```python
from build123d import *

# Parameters (mm, degrees)
SKETCH105_W     = 290
SKETCH105_H     = 290
PAD053_DEPTH    = 10
SKETCH106_R     = 5
SKETCH106_R_2   = 2.5
POCKET048_DEPTH = 10.001
SKETCH107_W     = 270
SKETCH107_H     = 270
SKETCH107_W_2   = 260
SKETCH107_H_2   = 260
PAD054_DEPTH    = 5


with BuildPart() as part:
    # Sketch105 → Pad053 (new body)
    with BuildSketch(Plane.XY):
        Rectangle(SKETCH105_W, SKETCH105_H)
    extrude(amount=-PAD053_DEPTH)

    # Sketch106 (on Face5 of Pad053) → Pocket048 (cut, through all)
    with BuildSketch(Plane.XY):
        with Locations((-120, 0)):
            Circle(SKETCH106_R)
        with Locations((0, 120)):
            Circle(SKETCH106_R)
        with Locations((120, 0)):
            Circle(SKETCH106_R)
        with Locations((0, -120)):
            Circle(SKETCH106_R)
        with Locations((0, 35.5)):
            Circle(SKETCH106_R_2)
    extrude(amount=-POCKET048_DEPTH, mode=Mode.SUBTRACT)

    # Sketch107 (on Face5 of Pocket048) → Pad054 (join)
    with BuildSketch(Plane(origin=(0, 0, -10), x_dir=(1, 0, 0), z_dir=(0, 0, -1))):
        Rectangle(SKETCH107_W, SKETCH107_H)
        Rectangle(SKETCH107_W_2, SKETCH107_H_2, mode=Mode.SUBTRACT)
    extrude(amount=PAD054_DEPTH)


with BuildPart() as part_1:
    # Body028 placement: moved
    add(part.part.moved(Location((0, 0, -10))))


solid = part_1.part
```
Source: CAD feature listing. Evaluate the final solid. Frame: model axes, mm. Give positions to 0.01 mm unless a question says otherwise; leave off trailing zeros. Loops run counter-clockwise (first coordinate to the right, second up) from the corner with the lowest first, then second, coordinate; pieces in that order, holes last. Notation, with made-up numbers: (39, 48) - (80, 48) arc R35 ccw to (80, 82) - close; hole circle Ø10 at (1, 19). An arc over 180 degrees is marked (long way). Use CSV: the item, a comma, the result in double quotes.
1) Line query: line 1 (X direction, y = -51, z = -24); line 2 (Y direction, x = 0, z = -18). Output: solid intervals per line, ascending.
Worked out:
line 1,"x = -135 to -130, 130 to 135"
line 2,"y = -145 to -125, -115 to 33, 38 to 115, 125 to 145"
2) Mould query, pull axis X, two halves, no side actions, for faces 1 (the flat face through (-145, -2, -15)), 2 (the flat face through (-2, 145, -15)), 3 (the flat face through (145, -2, -15)), 4 (the flat face through (-2, 2, -20)). Classes: +X half, -X half, draft (parallel to the pull), parting line (faces both ways), or undercut.
Worked out:
face 1,"-X half"
face 2,"draft"
face 3,"+X half"
face 4,"undercut"
3) Cut plane D-D (x = -30). Output: boundary loops of the cut face in (y, z).
Worked out:
outline,"(-145, -20) - (-135, -20) - (-135, -25) - (-130, -25) - (-130, -20) - (130, -20) - (130, -25) - (135, -25) - (135, -20) - (145, -20) - (145, -10) - (-145, -10) - close"
4) Cut plane C-C (y = 0). Output: boundary loops of the cut face in (x, z).
Worked out:
outline,"(-145, -20) - (-135, -20) - (-135, -25) - (-130, -25) - (-130, -20) - (-125, -20) - (-125, -10) - (-145, -10) - close; (-115, -20) - (115, -20) - (115, -10) - (-115, -10) - close; (125, -20) - (130, -20) - (130, -25) - (135, -25) - (135, -20) - (145, -20) - (145, -10) - (125, -10) - close"
5) Pin query (flat end, axial travel): P1, Ø4, axis at x = 0, y = 35.5, coming from the +Z side; P2, Ø4, axis at y = -23.5, z = -23, coming from the -X side; P3, Ø3, axis at x = -109, y = -63.5, coming from the -Z side; P4, Ø2.5, axis at y = 61, z = -23, coming from the +X side. Return the tip coordinate at first contact, or that it passes through.
Worked out:
P1,"passes through"
P2,"stops at x = -135"
P3,"stops at z = -20"
P4,"stops at x = 135"
6) Cut plane A-A (y = -120). Output: boundary loops of the cut face in (x, z), and give its area (3 significant figures).
Worked out:
outline,"(-145, -20) - (-135, -20) - (-135, -25) - (-130, -25) - (-130, -20) - (-5, -20) - (-5, -10) - (-145, -10) - close; (5, -20) - (130, -20) - (130, -25) - (135, -25) - (135, -20) - (145, -20) - (145, -10) - (5, -10) - close"
area,"2,850 mm^2"
